Solid Edge part; units mm, degrees
sketch "Sketch1" plane through (0, 0, 0) normal (0, 0, 1) x (1, 0, 0)
  line L0 (-40, -50) -> (40, -50)
  line L1 (40, -50) -> (50, -50)
  line L2 (50, -50) -> (50, -40)
  line L3 (50, -40) -> (50, 40)
  line L4 (50, 50) -> (50, 40)
  line L5 (40, 50) -> (50, 50)
  line L6 (40, 50) -> (-40, 50)
  line L7 (-50, 50) -> (-40, 50)
  line L8 (-50, 40) -> (-50, 50)
  line L9 (-50, 40) -> (-50, -40)
  line L10 (-50, -40) -> (-50, -50)
  line L11 (-50, -50) -> (-40, -50)
extrude "Protrusion1" add sketch "Sketch1" against normal blind 5
sketch "Sketch2" plane through (0, 0, 0) normal (0, 0, 1) x (1, 0, 0)
  line L0 (50, 50) -> (40, 50)
  line L1 (40, 46) -> (40, 50)
  line L2 (40, 46) -> (46, 46)
  line L3 (46, 46) -> (46, 40)
  line L4 (46, 40) -> (50, 40)
  line L5 (50, 40) -> (50, 50)
  line L6 (50, -40) -> (50, -50)
  line L7 (50, -50) -> (40, -50)
  line L8 (40, -46) -> (40, -50)
  line L9 (46, -46) -> (40, -46)
  line L10 (46, -40) -> (46, -46)
  line L11 (46, -40) -> (50, -40)
  line L12 (-50, -50) -> (-40, -50)
  line L13 (-40, -46) -> (-40, -50)
  line L14 (-46, -46) -> (-40, -46)
  line L15 (-46, -40) -> (-46, -46)
  line L16 (-50, -40) -> (-46, -40)
  line L17 (-50, -40) -> (-50, -50)
  line L18 (-46, 40) -> (-46, 46)
  line L19 (-46, 46) -> (-40, 46)
  line L20 (-40, 46) -> (-40, 50)
  line L21 (-40, 50) -> (-50, 50)
  line L22 (-50, 50) -> (-50, 40)
  line L23 (-50, 40) -> (-46, 40)
  dimension "D1" = 40
  dimension "D2" = 40
  dimension "D3" = 50
  dimension "D4" = 50
  dimension "D5" = 50
  dimension "D6" = 50
  dimension "D7" = 40
  dimension "D8" = 46
  dimension "D9" = 46
  dimension "D10" = 50
  dimension "D11" = 50
  dimension "D12" = 40
  dimension "D13" = 50
  dimension "D14" = 50
  dimension "D15" = 50
  dimension "D16" = 40
extrude "ExtrudedCutout_1" cut sketch "Sketch2" against normal blind 11.3526
sketch "Sketch3" plane through (0, 0, 0) normal (0, 0, 1) x (1, 0, 0)
  circle A0 centre (-40, -42.86) radius 1.5
  circle A1 centre (-36.13, 42.87) radius 1.5
  circle A2 centre (40, -42.86) radius 1.5
  circle A3 centre (37.53, 42.87) radius 1.5
extrude "Cutout1" cut sketch "Sketch3" against normal blind 5
sketch "Sketch4" plane through (0, 0, 0) normal (0, 0, 1) x (0, 1, 0)
  line L0 (36.87, 44) -> (-36.86, 44)
  line L1 (-36.86, 44) -> (-36.86, 34)
  line L2 (-36.86, 34) -> (-44, 34)
  line L3 (-44, 34) -> (-44, -34)
  line L4 (-44, -34) -> (-36.86, -34)
  line L5 (-36.86, -34) -> (-36.86, -44)
  line L6 (-36.86, -44) -> (36.87, -44)
  line L7 (36.87, -44) -> (36.87, -31.53)
  line L8 (36.87, -31.53) -> (44, -31.53)
  line L9 (44, -31.53) -> (44, 30.13)
  line L10 (44, 30.13) -> (36.87, 30.13)
  line L11 (36.87, 30.13) -> (36.87, 44)
extrude "Cutout2" cut sketch "Sketch4" against normal blind 5
sketch "Sketch5" plane through (0, 0, 0) normal (0, 0, 1) x (1, 0, 0)
  circle A0 centre (-26.5, 35) radius 1.5
  circle A1 centre (31.5, 35) radius 1.5
  circle A2 centre (31.5, -14) radius 1.5
  circle A3 centre (-26.5, -14) radius 1.5
  line L0 (-44, 36.87) -> (-30.13, 36.87)
  line L1 (-30.13, 38.87) -> (-30.13, 36.87)
  line L2 (31.53, 38.87) -> (-30.13, 38.87)
  line L3 (31.53, 38.87) -> (31.53, 36.87)
  line L4 (31.53, 36.87) -> (44, 36.87)
  line L5 (44, 36.87) -> (44, 32)
  line L6 (-44, 32) -> (44, 32)
  line L7 (-44, 35) -> (-44, 32)
  line L8 (-44, 35) -> (-44, 36.87)
  line L9 (-44, -14) -> (-44, -11)
  line L10 (-44, -11) -> (44, -11)
  line L11 (44, -11) -> (44, -17)
  line L12 (44, -17) -> (-44, -17)
  line L13 (-44, -17) -> (-44, -14)
  dimension "D1" = 26.5
extrude "ExtrudedProtrusion_2" add sketch "Sketch5" against normal blind 5
sketch "Sketch6" plane through (0, 0, 0) normal (0, 0, 1) x (1, 0, 0)
  line L0 (-46, 40) -> (-44, 40)
  line L1 (-44, 40) -> (-44, 46)
  line L2 (-44, 46) -> (-46, 46)
  line L3 (-46, 40) -> (-46, 46)
  line L4 (46, 46) -> (44, 46)
  line L5 (44, 46) -> (44, 40)
  line L6 (44, 40) -> (46, 40)
  line L7 (46, 40) -> (46, 46)
  line L8 (-46, -40) -> (-44, -40)
  line L9 (-44, -40) -> (-44, -46)
  line L10 (-44, -46) -> (-46, -46)
  line L11 (-46, -46) -> (-46, -40)
  line L12 (46, -46) -> (44, -46)
  line L13 (44, -46) -> (44, -40)
  line L14 (44, -40) -> (46, -40)
  line L15 (46, -40) -> (46, -46)
extrude "ExtrudedProtrusion_3" add sketch "Sketch6" along normal blind 5
sketch "Sketch7" plane through (-44, -43, 3) normal (1, 0, 0) x (0, 1, 0)
  circle A0 centre (0, -1) radius 1.5
  circle A1 centre (85.9991, -1) radius 1.5
extrude "ExtrudedCutout_14" cut sketch "Sketch7" against normal blind 2
sketch "Sketch8" plane through (44, 43, 2.5) normal (-1, 0, 0) x (0, -1, 0)
  circle A0 centre (0.0009, -0.5) radius 1.5
  circle A1 centre (86, -0.5) radius 1.5
extrude "ExtrudedCutout_15" cut sketch "Sketch8" against normal blind 2
fillet "Round_2" radius 1 8 edges at (45, 40, 5) (45, 46, 5) (-45, 40, 5) (-45, 46, 5) (-45, -46, 5) (-45, -40, 5) (45, -46, 5) (45, -40, 5)
Could you check a few things on this model? Use its own coordinates, in mm. A direction names the side the tool comes from. Give positions to 0.01 mm unless a question says otherwise; leave off trailing zeros. Order: outer loops, then holes, each group sorted by start corner. A loop starts at its lowest first (then second) coordinate and runs counter-clockwise, first axis right, second up.
Q1. Suppose I cut it at A-A, the plane x = -19. Write out the boundary of the cut face in (y, z), and give its area (3 significant figures).
Q2. I'm going to push flat-ended pins straight in: P1, Ø5.5, axis at y = -42, z = 3.5, coming from the -X side; P2, Ø3.5, axis at x = 37.53, y = 42.87, coming from the +Z side; P3, Ø3, axis at y = 43.5, z = 0.5, coming from the +X side. Where does each tip first touch, or does it pass through?
Q3. For faces 5 (the flat face through (39, -36.86, -2)), 6 (the flat face through (40, 48, -2)), 7 (the flat face through (-44, 46, -1)), 8 (the flat face through (-44, -43, 4)), which set-ups out of +Z, -Z, +X, -X, +Y, -Y let a thin tool reach every point of the face, with its end or its side?
Q4. We'd pull the mould along Y, two halves only. Please class faces 1 (the flat face through (-48, 40, -2)), 2 (the flat face through (34, -40, -2)), 3 (the cylindrical face through (-37.24, 43.88, -2.46)), 4 (the flat face through (46, 43, 0)): +Y half, -Y half, draft (parallel to the pull), parting line (faces both ways), or undercut.
Q5. If I drill on line 1 along Y through (x, z) = (37.53, -1.75); line 2 along Z through (x, y) = (-44.9, -43); line 3 along Y through (x, z) = (-12, -1.75), over which ranges is the centre line in solid material (lowest first)?
Q6. Suppose I cut it at B-B, the plane y = -3. Write out the boundary of the cut face in (x, z).
Q7. Suppose I cut it at C-C, the plane y = -14. Write out the boundary of the cut face in (x, z), and give its area (3 significant figures).
Solution:
1. outline: (-50, -5) - (-44, -5) - (-44, 0) - (-50, 0) - close; (-17, -5) - (-11, -5) - (-11, 0) - (-17, 0) - close; (32, -5) - (38.87, -5) - (38.87, 0) - (32, 0) - close; (44, -5) - (50, -5) - (50, 0) - (44, 0) - close
1. area: 124 mm2
2. P1: stops at x = -46
2. P2: stops at z = 0
2. P3: stops at x = 46
3. face 5: +Z, -Z
3. face 6: +Z, -Z, +X, +Y
3. face 7: +Z, -Z, -X, +Y
3. face 8: +Z, +Y, -Y
4. face 1: +Y half
4. face 2: undercut
4. face 3: undercut
4. face 4: draft
5. line 1: y = -50 to -36.86, -17 to -11, 32 to 41.37, 44.37 to 50
5. line 2: z = -5 to 0.5, 3.5 to 5
5. line 3: y = -50 to -44, -17 to -11, 32 to 38.87, 44 to 50
6. outline: (-50, -5) - (-44, -5) - (-44, 0) - (-50, 0) - close; (44, -5) - (50, -5) - (50, 0) - (44, 0) - close
7. outline: (-50, -5) - (-28, -5) - (-28, 0) - (-50, 0) - close; (-25, -5) - (30, -5) - (30, 0) - (-25, 0) - close; (33, -5) - (50, -5) - (50, 0) - (33, 0) - close
7. area: 470 mm2
